```python
from build123d import *

# Parameters (mm, degrees)
BOSS_EXTRUDE1_DEPTH  = 1.75
SKETCH3_R            = 0.675
CUT_EXTRUDE1_DEPTH   = 15
SKETCH4_R            = 0.675
CUT_EXTRUDE2_DEPTH   = 15
CUT_SWEEP1_START     = 1.740413317
CUT_SWEEP1_OUTLINE_R = 0.675
CUT_SWEEP1_DEPTH     = 15.070945459


# Read off the part's stored shape, not the designer's step: Cut-Sweep1
with BuildPart() as part:
    # Sketch2 → Boss-Extrude1 (new, symmetric)
    with BuildSketch(Plane(origin=(0, 0, 0), x_dir=(1, 0, 0), z_dir=(0, 1, 0))):
        Polygon((-1.271449424, 1.75), (-6.692503299, -14.934288264), (-3.363805492, -16.015847744), (1.271449424, -1.75), (16.271449424, -1.75), (16.271449424, 1.75), align=None)
    extrude(amount=BOSS_EXTRUDE1_DEPTH, both=True)

    # Sketch3 → Cut-Extrude1 (cut)
    with BuildSketch(Plane(origin=(-5.028154395, 0, 15.475068004), x_dir=(0.9510565162951536, 0, 0.3090169943749472), z_dir=(-0.3090169943749472, 0, 0.9510565162951536))):
        Circle(SKETCH3_R)
    extrude(amount=-CUT_EXTRUDE1_DEPTH, mode=Mode.SUBTRACT)

    # Sketch4 → Cut-Extrude2 (cut)
    with BuildSketch(Plane(origin=(16.271449424, 0, 0), x_dir=(0, 0, -1), z_dir=(1, 0, 0))):
        Circle(SKETCH4_R)
    extrude(amount=-CUT_EXTRUDE2_DEPTH, mode=Mode.SUBTRACT)

    # Sweep1: sweep along a path in Sketch7
    with BuildLine(Plane(origin=(0, 0, 0), x_dir=(0.7071067811865477, 0, 0.7071067811865475), z_dir=(-0.7071067811865475, 0, 0.7071067811865477))) as sweep1_path:
        Line((0, 1.75), (1.567926949, 16.667828431))
    # Sketch5 → Sweep1 (sweep)
    with BuildSketch(Plane(origin=(0, 1.75, 0), x_dir=(1, 0, 0), z_dir=(0, 1, 0))):
        Polygon((1.271449424, -1.75), (-2.408668361, -1.75), (-1.271449424, 1.75), (2.408668361, 1.75), align=None)
    sweep(path=sweep1_path.line)

    # Cut-Sweep1 outline → Cut-Sweep1 (cut)
    with BuildSketch(Plane(origin=(0, 0, 0), x_dir=(0.9972647091838012, -0.07370950015142784, -0.0054780839693199055), z_dir=(0.07391278520356448, 0.9945218953682737, 0.07391278520356448)).offset(CUT_SWEEP1_START)):
        with Locations((-0.128991625, 0.129702147)):
            Circle(CUT_SWEEP1_OUTLINE_R)
    extrude(amount=CUT_SWEEP1_DEPTH, mode=Mode.SUBTRACT)


solid = part.part
```
The listing builds one solid part. Answer for the finished solid, in the listing's coordinates (mm). A direction names the side the tool comes from. Coordinates: 2 decimals unless noted, no trailing zeros. Loops run counter-clockwise (first coordinate to the right, second up) from the corner with the lowest first, then second, coordinate; pieces in that order, holes last. Notation, with made-up numbers: M 62.25,2 L 76.25,2 A22 ccw 76.25,39 Z; hole C 4.25,-14 d10. An arc over 180 degrees is marked long. Answer as CSV lines item,"result". Start each with the question number.
(1) The mould has two halves that part along Z. Classify faces 1 (the flat face through (1.271, 0, 0)), 2 (the flat face through (16.271, 0, 1)), 3 (the flat face through (1.16, 9.31, -1.19)): pulls with the +Z half, pulls with the -Z half, needs draft (parallel to the pull), parting line crosses it, or undercut.
(2) The part is cut by section C-C (z = 2.5). State how many separate pieces and enclosed holes the cut face has, and give its area (3 significant figures).
(3) Find the intervals of material crossed by L1, parallel to Z at x = 15.25, y = 0.5; L2, parallel to X at y = 13.5, z = 0, in increasing order. Write a range as [from, to].
(4) For faces 4 (the cylindrical face through (8.88, -0.66, 0.15)), 5 (the flat face through (-0.01, 1.75, -0.01)), 6 (the flat face through (-0.05, 9.31, 2.31)), 7 (the flat face through (2.394, 9.313, 0.587)), 8 (the flat face through (2, 16.668, 1)), determine the directions among +Z, -Z, +X, -X, +Y, -Y from which every point of the face is accessible in a straight line to the end or side of a thin tool.
(5) The part is cut by section A-A (x = 12.5). Give the vertices of the cut face in (y, z) (3 decimals), and give its area (3 significant figures).
(6) Given pin 1 (1.5 mm diameter, centred on y = 10.5, z = 0.5, fed in from -X); pin 2 (3 mm diameter, centred on x = 11.5, z = 0.5, fed in from +Y); pin 3 (5 mm diameter, centred on x = 0.5, y = 7.5, fed in from +Z); pin 4 (1.5 mm diameter, centred on y = -0.5, z = 0, fed in from +X), each flat-ended and moving along its own axis, determine where each tip first touches the part or whether it passes through.
Determined:
1,face 1,"undercut"
1,face 2,"needs draft"
1,face 3,"pulls with the -Z half"
2,separate pieces,"2"
2,enclosed holes,"1"
2,area,"29.1 mm2"
3,L1,"[-1.75, -0.45], [0.45, 1.75]"
3,L2,"[-0.68, 3]"
4,face 4,"+X"
4,face 5,"none"
4,face 6,"+Z, +X, -X"
4,face 7,"+Z, +X"
4,face 8,"+Z, -Z, +X, -X, +Y"
5,outline,"M -1.75,-1.75 L 1.75,-1.75 L 1.75,1.75 L -1.75,1.75 Z; hole C 0,0 d1.35"
5,area,"10.8 mm2"
6,pin 1,"x = -1.4"
6,pin 2,"y = 1.75"
6,pin 3,"z = 2.36"
6,pin 4,"x = 16.27"
